from build123d import *

# Parameters (mm, degrees)
BOSS_EXTRUDE1_DEPTH = 30
SKETCH2_W           = 19.5
SKETCH2_H           = 3
BOSS_EXTRUDE2_DEPTH = 8
FILLET1_R           = 3
FILLET2_R           = 3
FILLET3_R           = 3
FILLET4_R           = 3


with BuildPart() as part:
    # Sketch1 → Boss-Extrude1 (new body)
    with BuildSketch(Plane.XY):
        Polygon((0, 0), (0, 22.5), (-19.5, 22.5), (-19.5, 19.5), (-3, 19.5), (-3, 3), (-19.5, 3), (-19.5, 0), align=None)
    extrude(amount=BOSS_EXTRUDE1_DEPTH)

    # Sketch2 → Boss-Extrude2 (add)
    with BuildSketch(Plane(origin=(0, 22.5, 0), x_dir=(1, 0, 0), z_dir=(0, 1, 0))):
        with Locations((-9.75, -5.25)):
            Rectangle(SKETCH2_W, SKETCH2_H)
        with Locations((-9.75, -24.75)):
            Rectangle(SKETCH2_W, SKETCH2_H)
    extrude(amount=BOSS_EXTRUDE2_DEPTH)

    # Fillet1
    fillet1_edges = [part.edges().sort_by_distance(p)[0] for p in [
        (-9.75, 30.5, 6.75),
    ]]
    fillet(fillet1_edges, radius=FILLET1_R - 0.0001)  # a hair under: the kernel refuses the full size

    # Fillet2
    fillet2_edges = [part.edges().sort_by_distance(p)[0] for p in [
        (-9.75, 30.5, 23.25),
    ]]
    fillet(fillet2_edges, radius=FILLET2_R - 0.0001)  # a hair under: the kernel refuses the full size

    # Fillet3
    fillet3_edges = [part.edges().sort_by_distance(p)[0] for p in [
        (-19.5, 19.5, 15),
    ]]
    fillet(fillet3_edges, radius=FILLET3_R - 0.0001)  # a hair under: the kernel refuses the full size

    # Fillet4
    fillet4_edges = [part.edges().sort_by_distance(p)[0] for p in [
        (-19.5, 3, 15),
    ]]
    fillet(fillet4_edges, radius=FILLET4_R - 0.0001)  # a hair under: the kernel refuses the full size


solid = part.part
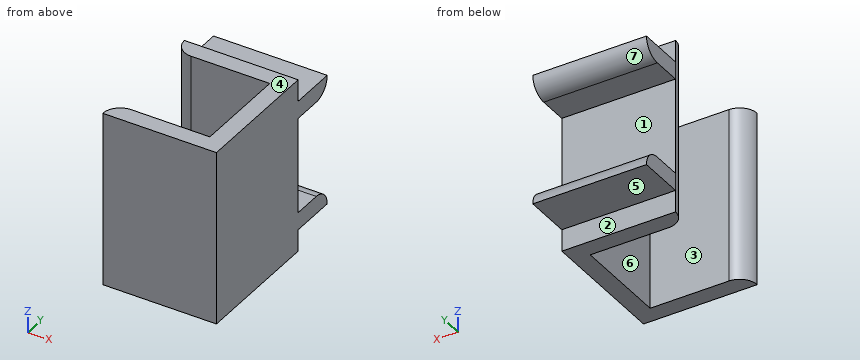
Model file for the job. Use its own axes, mm. Face numbers are marked on the shaded views. A direction names the side the tool comes from. Round coordinates to 2 decimals unless told otherwise and drop trailing zeros. Order: outer loops, then holes, each group sorted by start corner. A loop starts at its lowest first (then second) coordinate and runs counter-clockwise, first axis right, second up. Notation, with made-up numbers: M 13,-3.5 L 40,-3.5 A19 cw 40,25.5 Z; hole C -3,13 d10. An arc over 180 degrees is marked long. Write each question's results on one line, items separated by ' | '. Start each with the question number.
(1) Which spindle directions (+Z, -Z, +X, -X, +Y, -Y) get a long thin tool onto all of the face, cutting with end or side? Do the marked faces 1, 2 and 3. Say none if no direction does.
(2) Drop flat-ended pins along their axis: pin 1 (1.1 mm diameter, centred on x = -14, z = 1.5, fed in from +Y); pin 2 (5 mm diameter, centred on y = 10, z = 17.5, fed in from -X); pin 3 (1.5 mm diameter, centred on x = -9.5, y = 25, fed in from -Z); pin 4 (2 mm diameter, centred on y = 24.5, z = 10.5, fed in from -X). Give the stop position or say it passes through.
(3) Saw through at B-B, the plane y = 23. Give the cut face in (x, z).
(4) Saw through at D-D, the plane y = 4. Give the cut face in (x, z).
(5) Probe probe 1 along Y at (x, z) = (-14, 28.5); probe 2 along Z at (x, y) = (-1.5, 27); probe 3 along X at (y, z) = (9.5, 26.75). List the from-to ranges inside material, lowest first. Write a range as from..to.
(6) Two-plate mould, pull along Z, no slides. Class the marked faces 4, 5, 6 and 7: pulls with the +Z half, pulls with the -Z half, needs draft (parallel to the pull), parting line crosses it, or undercut.
Established:
1) face 1: +X, -X, +Y | face 2: -Z, +X, -X, +Y | face 3: +Z, -Z, -X
2) pin 1: stops at y = 22.5 | pin 2: stops at x = -3 | pin 3: stops at z = 3.75 | pin 4: passes through
3) outline: M -19.5,3.75 L 0,3.75 L 0,6.75 L -19.5,6.75 Z; M -19.5,23.25 L 0,23.25 L 0,26.25 L -19.5,26.25 Z
4) outline: M -3,0 L 0,0 L 0,30 L -3,30 Z
5) probe 1: y = 0..3, 19.5..22.5 | probe 2: z = 3.75..6.75, 23.25..26.25 | probe 3: x = -3..0
6) face 4: pulls with the +Z half | face 5: pulls with the -Z half | face 6: needs draft | face 7: undercut
